```python
from build123d import *

# Parameters (mm, degrees)
SKETCH1_R           = 30
BOSS_EXTRUDE1_DEPTH = 5
SKETCH2_R           = 19.5
BOSS_EXTRUDE2_DEPTH = 1
SKETCH3_R           = 17.5
BOSS_EXTRUDE3_DEPTH = 10
SKETCH5_R           = 2.05
CUT_EXTRUDE1_DEPTH  = 44.829214002
SKETCH6_R           = 3.6
CUT_EXTRUDE2_DEPTH  = 3.5
SKETCH9_R           = 5.5
CUT_EXTRUDE5_DEPTH  = 4
SKETCH7_R           = 12.025
CUT_EXTRUDE3_DEPTH  = 5
SKETCH8_R           = 10.5
CUT_EXTRUDE4_DEPTH  = 44.829214002


with BuildPart() as part:
    # Sketch1 → Boss-Extrude1 (new body)
    with BuildSketch(Plane.XY):
        Circle(SKETCH1_R)
    extrude(amount=BOSS_EXTRUDE1_DEPTH)

    # Sketch2 → Boss-Extrude2 (add)
    with BuildSketch(Plane.XY.offset(5)):
        Circle(SKETCH2_R)
    extrude(amount=BOSS_EXTRUDE2_DEPTH)

    # Sketch3 → Boss-Extrude3 (add)
    with BuildSketch(Plane.XY.offset(6)):
        Circle(SKETCH3_R)
    extrude(amount=BOSS_EXTRUDE3_DEPTH)

    # Sketch5 → Cut-Extrude1 (cut, through all)
    with BuildSketch(Plane.XY.offset(5)):
        with Locations((24.5, 0)):
            Circle(SKETCH5_R)
        with Locations((12.25, -21.217622393)):
            Circle(SKETCH5_R)
        with Locations((-12.25, -21.217622393)):
            Circle(SKETCH5_R)
        with Locations((-24.5, 0)):
            Circle(SKETCH5_R)
        with Locations((-12.25, 21.217622393)):
            Circle(SKETCH5_R)
        with Locations((12.25, 21.217622393)):
            Circle(SKETCH5_R)
    extrude(amount=-CUT_EXTRUDE1_DEPTH, mode=Mode.SUBTRACT)

    # Sketch6 → Cut-Extrude2 (cut)
    with BuildSketch(Plane.XY.offset(5)):
        with Locations((24.5, 0)):
            Circle(SKETCH6_R)
        with Locations((12.25, -21.217622393)):
            Circle(SKETCH6_R)
        with Locations((-12.25, -21.217622393)):
            Circle(SKETCH6_R)
        with Locations((-24.5, 0)):
            Circle(SKETCH6_R)
        with Locations((-12.25, 21.217622393)):
            Circle(SKETCH6_R)
        with Locations((12.25, 21.217622393)):
            Circle(SKETCH6_R)
    extrude(amount=-CUT_EXTRUDE2_DEPTH, mode=Mode.SUBTRACT)

    # Sketch9 → Cut-Extrude5 (cut)
    with BuildSketch(Plane(origin=(0, 0, 0), x_dir=(-1, 0, 0), z_dir=(0, 0, -1))):
        Circle(SKETCH9_R)
    extrude(amount=-CUT_EXTRUDE5_DEPTH, mode=Mode.SUBTRACT)

    # Sketch7 → Cut-Extrude3 (cut)
    with BuildSketch(Plane(origin=(0, 0, 0), x_dir=(-1, 0, 0), z_dir=(0, 0, -1))):
        Circle(SKETCH7_R)
    extrude(amount=-CUT_EXTRUDE3_DEPTH, mode=Mode.SUBTRACT)

    # Sketch8 → Cut-Extrude4 (cut, through all)
    with BuildSketch(Plane(origin=(0, 0, 5), x_dir=(-1, 0, 0), z_dir=(0, 0, -1))):
        Circle(SKETCH8_R)
    extrude(amount=-CUT_EXTRUDE4_DEPTH, mode=Mode.SUBTRACT)


solid = part.part
```
CAD build for the part. Positions are in the model's coordinates, mm. A direction names the side the tool comes from. Coordinates: 2 decimals unless noted, no trailing zeros. Write each loop counter-clockwise with the first axis right and the second up, starting at its lowest first coordinate (ties: lowest second). Pieces come first, ordered by that corner, then holes.
(1) Cut at D-D, the plane y = -22. List the corners of the cut face in (x, z).
(2) Drill centre lines: probe 1 along Y at (x, z) = (0, 11.5); probe 2 along X at (y, z) = (-20, 3.25); probe 3 along X at (y, z) = (-21, 2.25). Where is each one in solid material? Low to high.
(3) Flat gauge pins, fed straight in: pin 1 (3.5 mm diameter, centred on x = 25, y = -1, fed in from +Z); pin 2 (1.5 mm diameter, centred on y = 7.5, z = 13.5, fed in from -X); pin 3 (1.5 mm diameter, centred on y = 4, z = 13.5, fed in from -X); pin 4 (12.5 mm diameter, centred on x = 0, y = 0, fed in from +Z). Where does each tip first touch, or does it go through?
(4) Cut at C-C, the plane z = 14. List the corners of the cut face in (x, y), and give its area (3 significant figures).
(5) Two-plate mould, pull along Y, no slides. Class faces 1 (the face through (10.6, 20, 0.8)), 2 (the face through (0, -13, 0)), 3 (the face through (-29.97, 1.32, 2.46)): +Y half, -Y half, draft (parallel to the pull), parting line (faces both ways), or undercut.
(6) Cut at B-B, the plane y = 0. Count the separate pieces of the cut face and the enclosed holes in it, and give its area (3 significant figures).
(7) 3-axis set-ups, long thin cutter, end or side, ignore diameter. For faces 4 (the face through (0, -20, 5)), 5 (the face through (0, -11, 5)), 6 (the face through (-13.76, -19.83, 0.76)): which of +Z, -Z, +X, -X, +Y, -Y reach the whole face in a straight line?
(8) Cut at A-A, the plane x = 0. List the corners of the cut face in (y, z) (3 decimals), and give its area (3 significant figures).
Geometry says:
1. outline: (-20.4, 0) - (-14.14, 0) - (-14.14, 1.5) - (-15.76, 1.5) - (-15.76, 5) - (-20.4, 5) - close; (-10.36, 0) - (10.36, 0) - (10.36, 1.5) - (8.74, 1.5) - (8.74, 5) - (-8.74, 5) - (-8.74, 1.5) - (-10.36, 1.5) - close; (14.14, 0) - (20.4, 0) - (20.4, 5) - (15.76, 5) - (15.76, 1.5) - (14.14, 1.5) - close
2. probe 1: y = -17.5 to -10.5, 10.5 to 17.5
2. probe 2: x = -22.36 to -15.64, -8.86 to 8.86, 15.64 to 22.36
2. probe 3: x = -21.42 to -15.84, -8.66 to 8.66, 15.84 to 21.42
3. pin 1: stops at z = 1.5
3. pin 2: stops at x = -16.15
3. pin 3: stops at x = -17.2
3. pin 4: passes through
4. outline: circle Ø35 at (0, 0); hole circle Ø21 at (0, 0)
4. area: 616 mm2
5. face 1: undercut
5. face 2: draft
5. face 3: parting line
6. separate pieces: 4
6. enclosed holes: 0
6. area: 275 mm2
7. face 4: +Z
7. face 5: -Z
7. face 6: +Z, -Z
8. outline: (-30, 0) - (-12.025, 0) - (-12.025, 5) - (-10.5, 5) - (-10.5, 16) - (-17.5, 16) - (-17.5, 6) - (-19.5, 6) - (-19.5, 5) - (-30, 5) - close; (10.5, 5) - (12.025, 5) - (12.025, 0) - (30, 0) - (30, 5) - (19.5, 5) - (19.5, 6) - (17.5, 6) - (17.5, 16) - (10.5, 16) - close
8. area: 338 mm2
